Work out the finished part from the listing and answer in its coordinate system (mm). Face numbers are marked on the shaded views. Give positions to 0.01 mm unless a question says otherwise; leave off trailing zeros. Order: outer loops, then holes, each group sorted by start corner. A loop starts at its lowest first (then second) coordinate and runs counter-clockwise, first axis right, second up. Notation, with made-up numbers: M -16.75,-28 L 4.25,-28 A15 cw 4.25,-6 Z; hole C -1,81 d7. An arc over 180 degrees is marked long. One line per item, written item: value.
Autodesk Inventor part; units mm, degrees
ref_plane "YZ Plane" through (0, 0, 0) normal (1, 0, 0) x (0, 1, 0)
ref_plane "XZ Plane" through (0, 0, 0) normal (0, 1, 0) x (-1, 0, 0)
ref_plane "XY Plane" through (0, 0, 0) normal (0, 0, 1) x (1, 0, 0)
sketch "Sketch1" plane through (0, 0, 0) normal (1, 0, 0) x (0, 1, 0)
  circle A0 centre (0, 0) radius 11
  line L0 (0, 0) -> (0, -12.7) construction
  line L1 (0, -12.7) -> (6.35, -12.7) construction
  circle A1 centre (6.35, -12.7) radius 1.7526
  circle A2 centre (-6.35, -12.7) radius 1.7526
  circle A3 centre (6.35, 12.7) radius 1.7526
  circle A4 centre (-6.35, 12.7) radius 1.7526
  line L2 (12.7, 15.875) -> (-12.7, 15.875)
  line L3 (-12.7, 15.875) -> (-12.7, -15.875)
  line L4 (-12.7, -15.875) -> (12.7, -15.875)
  line L5 (12.7, -15.875) -> (12.7, 15.875)
  line L6 (12.7, 15.875) -> (-12.7, -15.875) construction
  line L7 (-12.7, 15.875) -> (12.7, -15.875) construction
  line L8 (0, 0) -> (9, 0) construction
  dimension "d0" = 22
  dimension "d1" = 12.7
  dimension "d2" = 6.35
  dimension "d3" = 3.5052
  dimension "d6" = 12.7
  dimension "d9" = 25.4
  dimension "d12" = 25.4
  dimension "d13" = 31.75
  dimension "d15" = 9
extrude "Extrusion1" add sketch "Sketch1" along normal blind 3.175
fillet "Fillet1" radius 3.175 4 edges at (1.5875, 12.7, 15.875) (1.5875, -12.7, 15.875) (1.5875, 12.7, -15.875) (1.5875, -12.7, -15.875)
equation "\"d9\" = 2 * d1"
properties part number "Motor Plates" material "UHMW, Black"
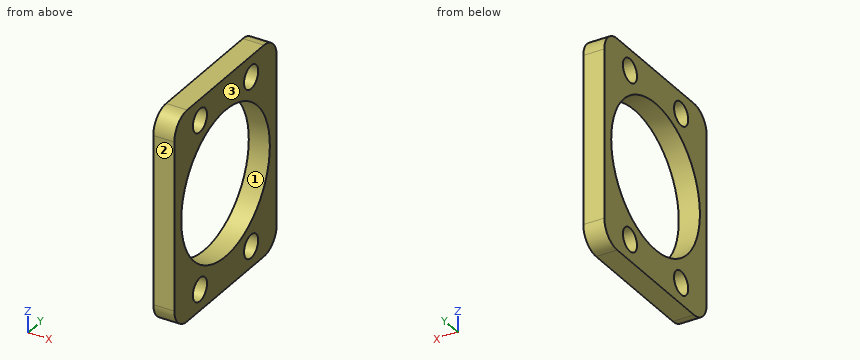
(1) Section A-A, the plane z = 0 is taken. Give the vertices of the cut face in (x, y) (3 decimals), then the cut area to 3 significant figures.
Findings:
outline: M 0,-12.7 L 3.175,-12.7 L 3.175,-11 L 0,-11 Z; M 0,11 L 3.175,11 L 3.175,12.7 L 0,12.7 Z
area: 10.8 mm^2
(2) Given P1, Ø3, axis at y = 6.35, z = -12.7, coming from the +X side, flat-ended and moving along its own axis, determine where the tip first touches the part or whether it passes through.
Findings:
P1: passes through
(3) Find the intervals of material crossed by probe 1 along Z at (x, y) = (0.3, 1) (3 decimals); probe 2 along Z at (x, y) = (0.4, 6.25) (3 decimals); probe 3 along Z at (x, y) = (2, 6.35) (3 decimals), in increasing order. Write a range as from..to.
Findings:
probe 1: z = -15.875..-10.954, 10.954..15.875
probe 2: z = -15.875..-14.45, -10.95..-9.052, 9.052..10.95, 14.45..15.875
probe 3: z = -15.875..-14.453, -10.947..-8.982, 8.982..10.947, 14.453..15.875
(4) Section B-B, the plane x = 2 is taken. Give the vertices of the cut face in (y, z) (3 decimals), then the cut area to 3 significant figures.
Findings:
outline: M -12.7,-12.7 A3.175 ccw -9.525,-15.875 L 9.525,-15.875 A3.175 ccw 12.7,-12.7 L 12.7,12.7 A3.175 ccw 9.525,15.875 L -9.525,15.875 A3.175 ccw -12.7,12.7 Z; hole C 0,0 d22; hole C -6.35,-12.7 d3.505; hole C -6.35,12.7 d3.505; hole C 6.35,-12.7 d3.505; hole C 6.35,12.7 d3.505
area: 379 mm^2
(5) Section D-D, the plane y = 6.35 is taken. Give the vertices of the cut face in (x, z) (3 decimals).
Findings:
outline: M 0,-15.875 L 3.175,-15.875 L 3.175,-14.453 L 0,-14.453 Z; M 0,-10.947 L 3.175,-10.947 L 3.175,-8.982 L 0,-8.982 Z; M 0,8.982 L 3.175,8.982 L 3.175,10.947 L 0,10.947 Z; M 0,14.453 L 3.175,14.453 L 3.175,15.875 L 0,15.875 Z
(6) Determine the mould class of the marked faces 1, 2 and 3 for opening direction Y: pulls with the +Y half, pulls with the -Y half, needs draft (parallel to the pull), parting line crosses it, or undercut.
Findings:
face 1: undercut
face 2: pulls with the -Y half
face 3: needs draft
(7) Section C-C, the plane y = 0 is taken. Give the vertices of the cut face in (x, z) (3 decimals), then the cut area to 3 significant figures.
Findings:
outline: M 0,-15.875 L 3.175,-15.875 L 3.175,-11 L 0,-11 Z; M 0,11 L 3.175,11 L 3.175,15.875 L 0,15.875 Z
area: 31.0 mm^2
